For this review, use the dimensioned drawing (mm, ordinates from the lowest corner) and the shaded views. Coordinates: 2 decimals unless noted, no trailing zeros. Loops run counter-clockwise (first coordinate to the right, second up) from the corner with the lowest first, then second, coordinate; pieces in that order, holes last. Notation, with made-up numbers: M 28,19 L 41,19 A25 ccw 41,44 Z; hole C 64,15.25 d5. An arc over 180 degrees is marked long. One line per item, written item: value.
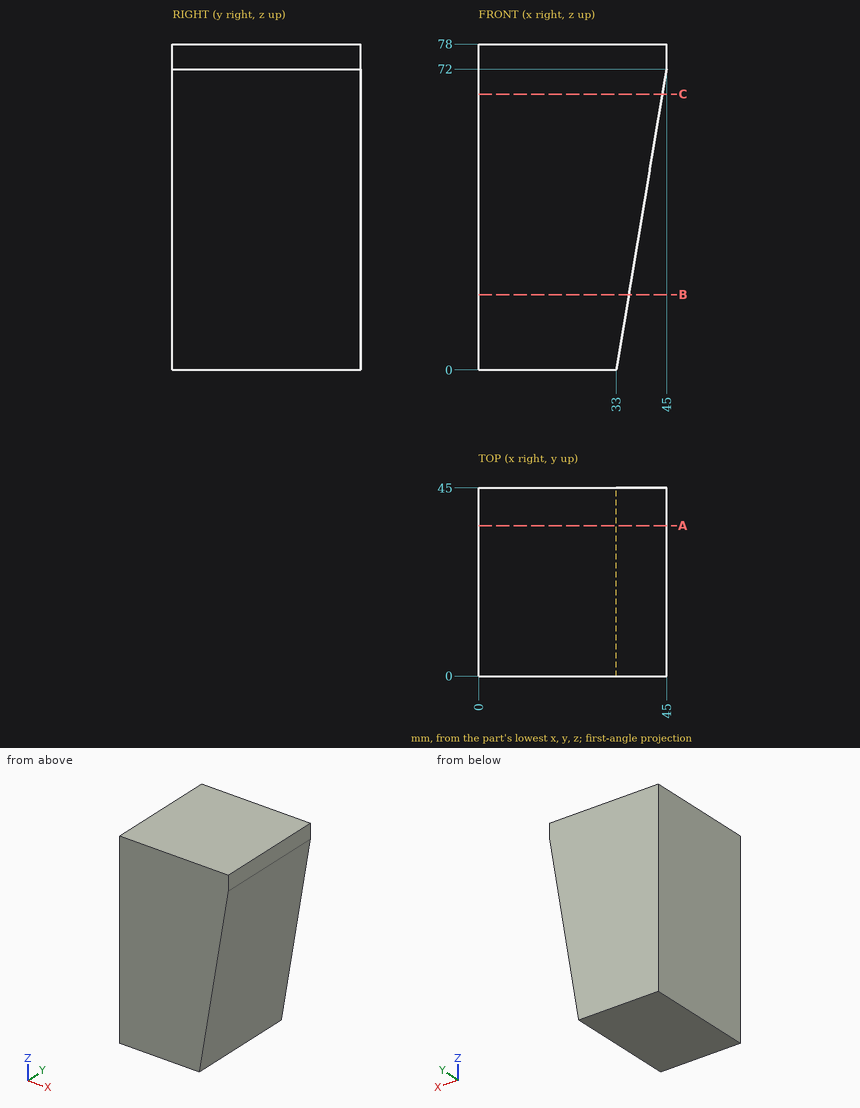
(1) To check wall thickness, follow L1, parallel to X at y = 37.5, z = 59; L2, parallel to X at y = 21.5, z = 8. State the ranges of each line that lie inside material, in increasing order. Write a range as [from, to].
Checks:
L1: [0, 42.83]
L2: [0, 34.33]
(2) Insertion check: pin 1 Ø2 at (y, z) = (19.5, 17) entering from +X. The pin has a flat end and moves straight along its axis. Give the tip position at first contact, or say it passes through.
Checks:
pin 1: x = 36
(3) Add section C-C on z = 66. State the section outline as (x, y) points, then the cut area to 3 significant figures.
Checks:
outline: M 0,0 L 44,0 L 44,45 L 0,45 Z
area: 1,980 mm^2
(4) Add section B-B on z = 18. State the section outline as (x, y) points.
Checks:
outline: M 0,0 L 36,0 L 36,45 L 0,45 Z
(5) Add section A-A on y = 36. State the section outline as (x, z) points.
Checks:
outline: M 0,0 L 33,0 L 45,72 L 45,78 L 0,78 Z
